```python
from build123d import *

# Parameters (mm, degrees)
F2_DEPTH = 15
F3_R     = 1.75
F4_DEPTH = 23.001
F5_R     = 3
F6_DEPTH = 4.5
F8_DEPTH = 1.2


with BuildPart() as f2:
    # F1 (on Front) → F2 (new body)
    with BuildSketch(Plane.XZ):
        with BuildLine():
            Line((-82, 0), (-40.5, 0))
            ThreePointArc((-40.5, 0), (-39.792893, 0.292893), (-39.5, 1))
            Line((-39.5, 1), (-39.5, 13.5))
            ThreePointArc((-39.5, 13.5), (-39.207107, 14.207107), (-38.5, 14.5))
            Line((-38.5, 14.5), (-29.5, 14.5))
            ThreePointArc((-29.5, 14.5), (-28.792893, 14.792893), (-28.5, 15.5))
            Line((-28.5, 15.5), (-28.5, 15.68045))
            ThreePointArc((-28.5, 15.68045), (-28.207107, 16.387557), (-27.5, 16.68045))
            ThreePointArc((-27.5, 16.68045), (-26.792893, 16.973344), (-26.5, 17.68045))
            Line((-26.5, 17.68045), (-26.5, 17.860901))
            ThreePointArc((-26.5, 17.860901), (-26.207107, 18.568008), (-25.5, 18.860901))
            Line((-25.5, 18.860901), (-21, 18.860901))
            ThreePointArc((-21, 18.860901), (-20.292893, 18.568008), (-20, 17.860901))
            Line((-20, 17.860901), (-20, 17.68045))
            ThreePointArc((-20, 17.68045), (-19.707107, 16.973344), (-19, 16.68045))
            ThreePointArc((-19, 16.68045), (-18.292893, 16.387557), (-18, 15.68045))
            Line((-18, 15.68045), (-18, 15.5))
            ThreePointArc((-18, 15.5), (-17.707107, 14.792893), (-17, 14.5))
            Line((-17, 14.5), (0, 14.5))
            Line((0, 14.5), (17, 14.5))
            ThreePointArc((17, 14.5), (17.707107, 14.792893), (18, 15.5))
            Line((18, 15.5), (18, 15.68045))
            ThreePointArc((18, 15.68045), (18.292893, 16.387557), (19, 16.68045))
            ThreePointArc((19, 16.68045), (19.707107, 16.973344), (20, 17.68045))
            Line((20, 17.68045), (20, 17.860901))
            ThreePointArc((20, 17.860901), (20.292893, 18.568008), (21, 18.860901))
            Line((21, 18.860901), (25.5, 18.860901))
            ThreePointArc((25.5, 18.860901), (26.207107, 18.568008), (26.5, 17.860901))
            Line((26.5, 17.860901), (26.5, 17.68045))
            ThreePointArc((26.5, 17.68045), (26.792893, 16.973344), (27.5, 16.68045))
            ThreePointArc((27.5, 16.68045), (28.207107, 16.387557), (28.5, 15.68045))
            Line((28.5, 15.68045), (28.5, 15.5))
            ThreePointArc((28.5, 15.5), (28.792893, 14.792893), (29.5, 14.5))
            Line((29.5, 14.5), (38.5, 14.5))
            ThreePointArc((38.5, 14.5), (39.207107, 14.207107), (39.5, 13.5))
            Line((39.5, 13.5), (39.5, 1))
            ThreePointArc((39.5, 1), (39.792893, 0.292893), (40.5, 0))
            Line((40.5, 0), (82, 0))
            Line((82, 0), (38, 23))
            Line((38, 23), (19.974391, 23))
            ThreePointArc((19.974391, 23), (10.263617, 19.399316), (0, 18.012873))
            ThreePointArc((0, 18.012873), (-10.263617, 19.399316), (-19.974391, 23))
            Line((-19.974391, 23), (-38, 23))
            Line((-38, 23), (-82, 0))
        make_face()
    extrude(amount=F2_DEPTH)

    # F3 (on Top) → F4 (cut, through all)
    with BuildSketch(Plane.XY):
        with Locations((66.75, -7.5)):
            Circle(F3_R)
        with Locations((-66.75, -7.5)):
            Circle(F3_R)
    extrude(amount=F4_DEPTH, mode=Mode.SUBTRACT)

    # F5 (on offset) → F6 (cut)
    with BuildSketch(Plane.XY.offset(10)):
        with Locations((-66.75, -7.505668)):
            Circle(F5_R)
        with Locations((66.75, -7.498881)):
            Circle(F5_R)
    extrude(amount=-F6_DEPTH, mode=Mode.SUBTRACT)

    # F7 (on Front) → F8 (join)
    with BuildSketch(Plane.XZ):
        with BuildLine():
            Line((-39.5, 13.5), (-39.5, 1.22279))
            Line((-39.5, 1.22279), (-29.826649, 14.5))
            Line((-29.826649, 14.5), (-38.5, 14.5))
            ThreePointArc((-38.5, 14.5), (-39.207107, 14.207107), (-39.5, 13.5))
        make_face()
        with BuildLine():
            Line((29.826649, 14.5), (39.5, 1.22279))
            Line((39.5, 1.22279), (39.5, 13.5))
            ThreePointArc((39.5, 13.5), (39.207107, 14.207107), (38.5, 14.5))
            Line((38.5, 14.5), (29.826649, 14.5))
        make_face()
    extrude(amount=F8_DEPTH)


solid = f2.part
```
Could you check a few things on this model? Use its own coordinates, in mm. A direction names the side the tool comes from. Give positions to 0.01 mm unless a question says otherwise; leave off trailing zeros. Write each loop counter-clockwise with the first axis right and the second up, starting at its lowest first coordinate (ties: lowest second). Pieces come first, ordered by that corner, then holes. Notation, with made-up numbers: (35.5, -18) - (87.5, -18) arc R19 ccw to (87.5, -10) - close; hole circle Ø1 at (15, 41). An arc over 180 degrees is marked (long way). One line per item, written item: value. Start each with the question number.
Item 1: Which directions (+Z, -Z, +X, -X, +Y, -Y) give clear straight access to the entire face, cutting with the end or side of a thin tool? Please do faces 4 (the face through (63.753, -7.367, 7.158)), 5 (the face through (-39.5, -7, 7)), 6 (the face through (-10.123, -7.395, 19.364)), 7 (the face through (0, -7, 14.5)).
Item 2: I'm going to push flat-ended pins straight in: pin 1 (1.5 mm diameter, centred on x = 25.5, y = -4, fed in from -Z); pin 2 (1.3 mm diameter, centred on x = -22.5, y = -9, fed in from -Z); pin 3 (2 mm diameter, centred on y = -8.5, z = 15.5, fed in from +X); pin 4 (8 mm diameter, centred on x = 18.5, z = 10, fed in from +Y). Where does each tip first touch, or does it pass through?
Item 3: Imagine slicing it at B-B, the plane x = -66.75. List the corners of the cut face in (y, z) for me, and give its area (3 significant figures).
Item 4: Please list where these lines run through material, in increasing order: line 1 (Y direction, x = 66.75, z = 7.4); line 2 (X direction, y = -14, z = 15.5); line 3 (Y direction, x = -66.75, z = 1.1). Write a range as from..to.
Item 5: Imagine slicing it at A-A, the plane z = 3.75. List the corners of the cut face in (x, y) for me, and give its area (3 significant figures).
Item 6: If we mould it in two halves opening along Y, with no side actions, what happens to faces 1 (the face through (-63.89, -6.6, 7.1)), 2 (the face through (-1, 0, 17)), 3 (the face through (-23, -7, 18.861))? For each: +Y half, -Y half, draft (parallel to the pull), parting line (faces both ways), or undercut.
Item 7: Imagine slicing it at C-C, the plane x = -45. List the corners of the cut face in (y, z) for me, and give its area (3 significant figures).
Geometry says:
1. face 4: +Z
1. face 5: -Z, -Y
1. face 6: +Z, +Y, -Y
1. face 7: -Z, +Y, -Y
2. pin 1: z = 18.52
2. pin 2: z = 18.86
2. pin 3: x = 54.26
2. pin 4: through
3. outline: (-15, 0) - (-9.25, 0) - (-9.25, 5.5) - (-10.51, 5.5) - (-10.51, 7.97) - (-15, 7.97) - close; (-5.75, 0) - (0, 0) - (0, 7.97) - (-4.51, 7.97) - (-4.51, 5.5) - (-5.75, 5.5) - close
3. area: 85.5 mm^2
4. line 1: -15..-10.5, -4.5..0
4. line 2: -52.35..-28.5, -18..18, 28.5..52.35
4. line 3: -15..-9.25, -5.75..0
5. outline: (-74.83, -15) - (-39.5, -15) - (-39.5, -1.2) - (-37.66, -1.2) - (-37.66, 0) - (-74.83, 0) - close; (37.66, -1.2) - (39.5, -1.2) - (39.5, -15) - (74.83, -15) - (74.83, 0) - (37.66, 0) - close; hole circle Ø3.5 at (-66.75, -7.5); hole circle Ø3.5 at (66.75, -7.5)
5. area: 1,040 mm^2
6. face 1: undercut
6. face 2: +Y half
6. face 3: draft
7. outline: (-15, 0) - (0, 0) - (0, 19.34) - (-15, 19.34) - close
7. area: 290 mm^2
